```python
from build123d import *

# Parameters (mm, degrees)
EXTRUDE_THIN1_DEPTH          = 245.284098
CUT_EXTRUDE1_DEPTH           = 248.90040083
SKETCH4_R                    = 6.35
CUT_EXTRUDE2_DEPTH           = 237.025978745
CUT_EXTRUDE3_DEPTH           = 251.811121627
F_1_8_0_135_DIAMETER_HOLE1_D = 3.429


with BuildPart() as part:
    # Sketch1 → Extrude-Thin1 (new body)
    with BuildSketch(Plane.XY):
        with BuildLine():
            Line((-12.7, 22.86), (-12.7, -22.86))
            ThreePointArc((-12.7, -22.86), (-11.956051224, -24.656051224), (-10.16, -25.4))
            Line((-10.16, -25.4), (10.16, -25.4))
            ThreePointArc((10.16, -25.4), (11.956051224, -24.656051224), (12.7, -22.86))
            Line((12.7, -22.86), (12.7, 22.86))
            ThreePointArc((12.7, 22.86), (11.956051224, 24.656051224), (10.16, 25.4))
            Line((10.16, 25.4), (-10.16, 25.4))
            ThreePointArc((-10.16, 25.4), (-11.956051224, 24.656051224), (-12.7, 22.86))
        make_face()
        with BuildLine():
            Line((-11.1125, 22.86), (-11.1125, -22.86))
            ThreePointArc((-11.1125, -22.86), (-10.833519209, -23.533519209), (-10.16, -23.8125))
            Line((-10.16, -23.8125), (10.16, -23.8125))
            ThreePointArc((10.16, -23.8125), (10.833519209, -23.533519209), (11.1125, -22.86))
            Line((11.1125, -22.86), (11.1125, 22.86))
            ThreePointArc((11.1125, 22.86), (10.833519209, 23.533519209), (10.16, 23.8125))
            Line((10.16, 23.8125), (-10.16, 23.8125))
            ThreePointArc((-10.16, 23.8125), (-10.833519209, 23.533519209), (-11.1125, 22.86))
        make_face(mode=Mode.SUBTRACT)
    extrude(amount=EXTRUDE_THIN1_DEPTH)

    # Sketch2 → Cut-Extrude1 (cut, through all)
    with BuildSketch(Plane(origin=(12.7, 0, 0), x_dir=(0, 0, -1), z_dir=(1, 0, 0))):
        Polygon((-245.284097937, 25.4), (-194.484097937, -25.4), (-245.284097937, -25.4), align=None)
        Polygon((0, 25.4), (-50.8, -25.4), (0, -25.4), align=None)
    extrude(amount=-CUT_EXTRUDE1_DEPTH, mode=Mode.SUBTRACT)

    # Sketch4 → Cut-Extrude2 (cut, through all)
    with BuildSketch(Plane(origin=(0, 12.7, 12.7), x_dir=(1, 0, 0), z_dir=(0, -0.7071067811865476, -0.7071067811865476))):
        with Locations((0, -22.318463274)):
            Circle(SKETCH4_R)
        with Locations(Location((0, -6.443463274, 0), (0, 0, 270))):
            Circle(SKETCH4_R)
        with Locations((0, -38.193463274)):
            Circle(SKETCH4_R)
    extrude(amount=-CUT_EXTRUDE2_DEPTH, mode=Mode.SUBTRACT)

    # Sketch5 → Cut-Extrude3 (cut, through all)
    with BuildSketch(Plane(origin=(0, 25.4, 0), x_dir=(1, 0, 0), z_dir=(0, 1, 0))):
        with BuildLine():
            Line((-6.35, -16.28756685), (-6.35, 0))
            Line((-6.35, 0), (6.35, 0))
            Line((6.35, 0), (6.35, -16.28756685))
            add(Edge.make_bspline(
                [(-6.35, -16.28756685), (-6.35, -25.267822971), (0, -25.267822971), (6.35, -25.267822971), (6.35, -16.28756685)],
                knots=[1.570796327, 1.570796327, 1.570796327, 3.141592654, 3.141592654, 4.71238898, 4.71238898, 4.71238898], degree=2, weights=[1, 0.707106781, 1, 0.707106781, 1]))
        make_face()
    extrude(amount=-CUT_EXTRUDE3_DEPTH, mode=Mode.SUBTRACT)

    # 1/8 (0.135) Diameter Hole1 (through all)
    with Locations(Plane.ZY.offset(12.7)):
        with Locations((63.5, 16.497783942), (57.15, 5.499261314), (50.8, 16.497783942), (38.1, 16.497783942), (25.4, 16.497783942), (31.75, 5.499261314), (44.45, 5.499261314), (38.1, -5.499261314), (50.8, -5.499261314), (63.5, -5.499261314), (57.15, -16.497783942), (69.85, -16.497783942), (181.784097937, 16.497783942), (194.484097937, 16.497783942), (207.184097937, 16.497783942), (219.884097937, 16.497783942), (213.534097937, 5.499261314), (200.834097937, 5.499261314), (188.134097937, 5.499261314), (175.434097937, 5.499261314), (181.784097937, -5.499261314), (194.484097937, -5.499261314), (207.184097937, -5.499261314), (188.134097937, -16.497783942), (175.434097937, -16.497783942)):
            Hole(F_1_8_0_135_DIAMETER_HOLE1_D / 2)


solid = part.part
```
Source: CAD feature listing. Evaluate the final solid. Frame: model axes, mm. A direction names the side the tool comes from. Round coordinates to 2 decimals unless told otherwise and drop trailing zeros. Loops run counter-clockwise (first coordinate to the right, second up) from the corner with the lowest first, then second, coordinate; pieces in that order, holes last. Notation, with made-up numbers: M 42.25,-23 L 91.25,-23 A15 ccw 91.25,2 Z; hole C 65,6 d9. An arc over 180 degrees is marked long. Put each result on its own line as item: value.
(1) Section A-A, the plane z = 123. Return loops of the section in (x, y) (1 decimal), and give its area (3 significant figures).
Solutions:
outline: M -12.7,-22.9 A2.5 ccw -10.2,-25.4 L 10.2,-25.4 A2.5 ccw 12.7,-22.9 L 12.7,22.9 A2.5 ccw 10.2,25.4 L -10.2,25.4 A2.5 ccw -12.7,22.9 Z; hole M -11.1,-22.9 A1 ccw -10.2,-23.8 L 10.2,-23.8 A1 ccw 11.1,-22.9 L 11.1,22.9 A1 ccw 10.2,23.8 L -10.2,23.8 A1 ccw -11.1,22.9 Z
area: 227 mm²
(2) Pull-direction query (Z, two-part tool) for faces 3 (the face through (0, -23.812, 122)), 4 (the face through (-12.2, -1.8, 27.2)), 5 (the face through (11.348, 0.119, 220.003)); classes: released by +Z, released by -Z, zero draft, split by the parting line, or undercut.
Solutions:
face 3: zero draft
face 4: released by -Z
face 5: released by +Z
(3) First-contact query: pin 1 (1 mm diameter, centred on x = 4.5, z = 28.5, fed in from -Y); pin 2 (2.5 mm diameter, centred on y = 5.5, z = 44.45, fed in from +X); pin 3 (4.5 mm diameter, centred on y = 16.5, z = 219.88, fed in from -X); pin 4 (1.3 mm diameter, centred on y = 24.5, z = 8.5, fed in from +X). Flat tips, straight axial feed; report the tip coordinate or a pass-through.
Solutions:
pin 1: y = 23.81
pin 2: through
pin 3: x = -12.7
pin 4: x = 12.5
(4) Access query for faces 1 (the face through (0, 25.4, 121)), 2 (the face through (11.112, 0, 121)). Directions: +Z, -Z, +X, -X, +Y, -Y. A direction counts if a zero-diameter tool reaches every point of the face in a straight line with its end or side. Return the directions, or none.
Solutions:
face 1: +Z, -Z, +X, -X, +Y
face 2: +Z, -Z
(5) Ray query, line 1 (X direction, y = 18, z = 57); line 2 (Y direction, x = -10.25, z = 109.5); line 3 (Y direction, x = -12.05, z = 38.1). Return the intervals inside material, ascending. Write a range as [from, to].
Solutions:
line 1: [-12.7, -11.11], [11.11, 12.7]
line 2: [-25.4, -23.81], [23.81, 25.4]
line 3: [-12.7, -7.21], [-3.78, 14.78], [18.21, 24.56]
